For this review, take the finished solid that the model builds, in its own axes (mm). Face numbers are marked on the shaded views. A direction names the side the tool comes from. Give positions to 0.01 mm unless a question says otherwise; leave off trailing zeros. Loops run counter-clockwise (first coordinate to the right, second up) from the corner with the lowest first, then second, coordinate; pieces in that order, holes last. Notation, with made-up numbers: (47, -20) - (104, -20) arc R21 cw to (104, 10) - close; hole circle Ø3 at (15, 71.5). An arc over 180 degrees is marked (long way). Answer as CSV lines item,"result".
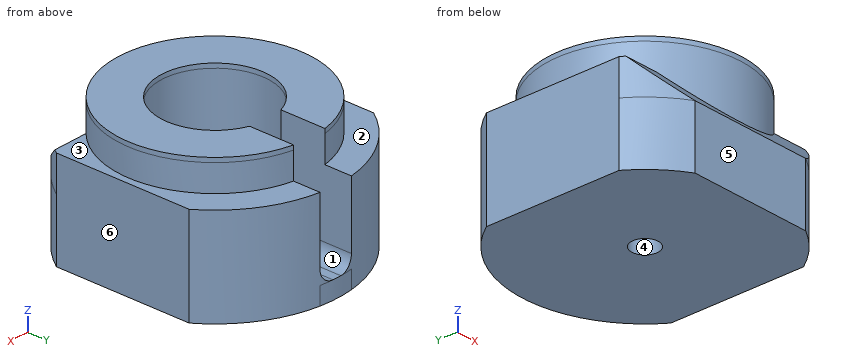
from build123d import *
from build123d.topology import SkipClean

# Parameters (mm, degrees)
SKETCH1_R               = 9.1
SKETCH1_R_2             = 6.1
BOSS_EXTRUDE1_DEPTH     = 12
BOSS_EXTRUDE2_START     = -3
SKETCH2_R               = 11
SKETCH2_R_2             = 9.1
BOSS_EXTRUDE2_DEPTH     = 3
BOSS_EXTRUDE3_START     = 4
SKETCH3_R               = 14
SKETCH3_R_2             = 11
SKETCH3_R_3             = 9.1
BOSS_EXTRUDE3_DEPTH     = 4
BOSS_EXTRUDE4_START     = 2
SKETCH4_R               = 9.1
SKETCH4_R_2             = 1.5
BOSS_EXTRUDE4_DEPTH     = 2
CUT_EXTRUDE3_DEPTH      = 23.649503306
CUT_EXTRUDE3_DEPTH_BACK = 23.649503306
SKETCH5_W               = 4
SKETCH5_H               = 12
CUT_EXTRUDE1_DEPTH      = 22.864640404
CUT_EXTRUDE4_DEPTH      = 22.864640404
CUT_EXTRUDE4_DEPTH_BACK = 22.864640404
SKETCH7_W               = 8
SKETCH7_H               = 10
BOSS_EXTRUDE5_START     = -14
SKETCH2_2_R             = 11
SKETCH2_2_R_2           = 9.1
SKETCH2_2_R_3           = 6.1
BOSS_EXTRUDE5_DEPTH     = 14
BOSS_EXTRUDE6_START     = 7
BOSS_EXTRUDE6_DEPTH     = 7
CUT_EXTRUDE5_START      = 5.762811814
CUT_EXTRUDE5_OUTLINE_W  = 4
CUT_EXTRUDE5_OUTLINE_H  = 12
CUT_EXTRUDE5_DEPTH      = 5.237188186
BOSS_EXTRUDE7_START     = -2
SKETCH11_R              = 14
SKETCH11_R_2            = 1.5
BOSS_EXTRUDE7_DEPTH     = 2
CUT_EXTRUDE6_DEPTH      = 24.151673806
CUT_EXTRUDE6_DEPTH_BACK = 24.151673806
FILLET1_R               = 1.5
BOSS_EXTRUDE8_DEPTH     = 0.5


# Read off the part's stored shape, not the designer's step: Cut-Extrude5
with BuildPart() as part:
    # Sketch1 → Boss-Extrude1 (new body)
    with BuildSketch(Plane.XY):
        Circle(SKETCH1_R)
        Circle(SKETCH1_R_2, mode=Mode.SUBTRACT)
    extrude(amount=BOSS_EXTRUDE1_DEPTH)

    # Sketch2 → Boss-Extrude2 (add)
    with BuildSketch(Plane.XY.offset(12).offset(BOSS_EXTRUDE2_START)):
        Circle(SKETCH2_R)
        Circle(SKETCH2_R_2, mode=Mode.SUBTRACT)
    extrude(amount=BOSS_EXTRUDE2_DEPTH)

    # Sketch3 → Boss-Extrude3 (add)
    # profile 1 of 2: a face of its own
    with BuildSketch(Plane(origin=(0, 0, 9), x_dir=(-1, 0, 0), z_dir=(0, 0, -1)).offset(BOSS_EXTRUDE3_START)):
        Circle(SKETCH3_R)
        with Locations(Location((0, 0, 0), (0, 0, 180))):
            Circle(SKETCH3_R_2, mode=Mode.SUBTRACT)
    # profile 2 of 2: a face of its own
    with BuildSketch(Plane(origin=(0, 0, 9), x_dir=(-1, 0, 0), z_dir=(0, 0, -1)).offset(BOSS_EXTRUDE3_START)):
        with Locations(Location((0, 0, 0), (0, 0, 180))):
            Circle(SKETCH3_R_2)
        Circle(SKETCH3_R_3, mode=Mode.SUBTRACT)
    extrude(amount=-BOSS_EXTRUDE3_DEPTH)

    # Sketch4 → Boss-Extrude4 (add)
    with BuildSketch(Plane(origin=(0, 0, 0), x_dir=(-1, 0, 0), z_dir=(0, 0, -1)).offset(BOSS_EXTRUDE4_START)):
        Circle(SKETCH4_R)
        Circle(SKETCH4_R_2, mode=Mode.SUBTRACT)
    extrude(amount=-BOSS_EXTRUDE4_DEPTH)

    # Sketch6 → Cut-Extrude3 (cut, two sides: drawn at the far end of the back side and taken through both)
    with BuildSketch(Plane.XY.offset(9).offset(-CUT_EXTRUDE3_DEPTH_BACK)):
        with BuildLine():
            ThreePointArc((11.75, -7.611668674), (14, 0), (11.75, 7.611668674))
            Line((11.75, 7.611668674), (11.75, -7.611668674))
        make_face()
        with BuildLine():
            Line((-11.75, -7.611668674), (-11.75, 7.611668674))
            ThreePointArc((-11.75, 7.611668674), (-14, 0), (-11.75, -7.611668674))
        make_face()
    extrude(amount=CUT_EXTRUDE3_DEPTH + CUT_EXTRUDE3_DEPTH_BACK, mode=Mode.SUBTRACT)

    # Sketch5 → Cut-Extrude1 (cut, through all)
    with BuildSketch(Plane(origin=(0, 0, 0), x_dir=(1, 0, 0), z_dir=(0, 1, 0))):
        with Locations((0, -6)):
            Rectangle(SKETCH5_W, SKETCH5_H)
    extrude(amount=CUT_EXTRUDE1_DEPTH, mode=Mode.SUBTRACT)

    # Sketch7 → Cut-Extrude4 (cut, two sides: drawn at the far end of the back side and taken through both)
    with BuildSketch(Plane(origin=(0, 0, 0), x_dir=(0, 0, -1), z_dir=(1, 0, 0)).offset(-CUT_EXTRUDE4_DEPTH_BACK)):
        with Locations((-8, -18.1)):
            Rectangle(SKETCH7_W, SKETCH7_H)
        Polygon((-12, -13.1), (-12, -6.1), (-12, -5.1), (-4, -13.1), align=None)
    extrude(amount=CUT_EXTRUDE4_DEPTH + CUT_EXTRUDE4_DEPTH_BACK, mode=Mode.SUBTRACT)

    # Sketch2<2> → Boss-Extrude5 (add)
    # profile 1 of 2: a face of its own
    with BuildSketch(Plane.XY.offset(12).offset(BOSS_EXTRUDE5_START)):
        Circle(SKETCH2_2_R)
        Circle(SKETCH2_2_R_2, mode=Mode.SUBTRACT)
    # profile 2 of 2: a face of its own
    with BuildSketch(Plane.XY.offset(12).offset(BOSS_EXTRUDE5_START)):
        Circle(SKETCH2_2_R_2)
        Circle(SKETCH2_2_R_3, mode=Mode.SUBTRACT)
    extrude(amount=BOSS_EXTRUDE5_DEPTH)

    # Sketch10 → Boss-Extrude6 (add)
    with BuildSketch(Plane(origin=(0, 0, 5), x_dir=(-1, 0, 0), z_dir=(0, 0, -1)).offset(BOSS_EXTRUDE6_START)):
        with BuildLine():
            Line((2, 13.856406461), (2, 10.816653826))
            ThreePointArc((2, 10.816653826), (0, -11), (-2, 10.816653826))
            Line((-2, 10.816653826), (-2, 13.856406461))
            ThreePointArc((-2, 13.856406461), (-7.550815354, 11.789197916), (-11.75, 7.611668674))
            Line((-11.75, 7.611668674), (-11.75, -7.611668674))
            ThreePointArc((-11.75, -7.611668674), (-9.660292592, -10.133052207), (-7.042016757, -12.1))
            Line((-7.042016757, -12.1), (7.042016757, -12.1))
            ThreePointArc((7.042016757, -12.1), (9.660292592, -10.133052207), (11.75, -7.611668674))
            Line((11.75, -7.611668674), (11.75, 7.611668674))
            ThreePointArc((11.75, 7.611668674), (7.550815354, 11.789197916), (2, 13.856406461))
        make_face()
    extrude(amount=-BOSS_EXTRUDE6_DEPTH)

    # Cut-Extrude5 outline → Cut-Extrude5 (cut)
    with BuildSketch(Plane(origin=(0, 0, 0), x_dir=(1, 0, 0), z_dir=(0, 1, 0)).offset(CUT_EXTRUDE5_START)):
        with Locations((0, -6)):
            Rectangle(CUT_EXTRUDE5_OUTLINE_W, CUT_EXTRUDE5_OUTLINE_H)
    extrude(amount=CUT_EXTRUDE5_DEPTH, mode=Mode.SUBTRACT)

    # Sketch11 → Boss-Extrude7 (add)
    with SkipClean():  # the faces are left unmerged after this step: merging them gives an invalid solid
        with BuildSketch(Plane.XY.offset(BOSS_EXTRUDE7_START)):
            with Locations(Location((0, 0, 0), (0, 0, 327.064769503))):
                Circle(SKETCH11_R)
            with Locations(Location((0, 0, 0), (0, 0, 180))):
                Circle(SKETCH11_R_2, mode=Mode.SUBTRACT)
        extrude(amount=BOSS_EXTRUDE7_DEPTH)

    # Sketch12 → Cut-Extrude6 (cut, two sides: drawn at the far end of the back side and taken through both)
    with SkipClean():  # the faces are left unmerged after this step: merging them gives an invalid solid
        with BuildSketch(Plane.XY.offset(-CUT_EXTRUDE6_DEPTH_BACK)):
            with BuildLine():
                Line((11.75, 7.611668674), (11.75, -7.611668674))
                ThreePointArc((11.75, -7.611668674), (14, 0), (11.75, 7.611668674))
            make_face()
            with BuildLine():
                Line((-11.75, -7.611668674), (-11.75, 7.611668674))
                ThreePointArc((-11.75, 7.611668674), (-14, 0), (-11.75, -7.611668674))
            make_face()
            with BuildLine():
                Line((7.042016757, -12.1), (-7.042016757, -12.1))
                ThreePointArc((-7.042016757, -12.1), (0, -14), (7.042016757, -12.1))
            make_face()
        extrude(amount=CUT_EXTRUDE6_DEPTH + CUT_EXTRUDE6_DEPTH_BACK, mode=Mode.SUBTRACT)

    # Fillet1
    # the kernel refuses this fillet: 1.5 mm, written as the material it adds along each edge
    with BuildSketch(Plane(origin=(-2, 2.012811814, 0), x_dir=(0, 0, 1), z_dir=(0, 1, 0))) as fillet1_piece_1_section:
        with BuildLine():
            CenterArc((FILLET1_R, FILLET1_R), FILLET1_R, 180, 90)
            Line((0, FILLET1_R), (0, 0))
            Line((0, 0), (FILLET1_R, 0))
        make_face()
    fillet1_piece_1 = extrude(amount=8.803842012, mode=Mode.PRIVATE)
    fillet1_piece_1 = fillet1_piece_1 - Plane(origin=(0, 0, 0.34289743), x_dir=(1, 0, 0), z_dir=(0, 0, -1)) * Cylinder(6.1, 24, mode=Mode.PRIVATE)
    add(fillet1_piece_1)
    with BuildSketch(Plane(origin=(2, 2.012811814, 0), x_dir=(0, 0, 1), z_dir=(0, 1, 0))) as fillet1_piece_2_section:
        with BuildLine():
            CenterArc((FILLET1_R, -FILLET1_R), FILLET1_R, 90, 90)
            Line((0, -FILLET1_R), (0, 0))
            Line((0, 0), (FILLET1_R, 0))
        make_face()
    fillet1_piece_2 = extrude(amount=8.803842012, mode=Mode.PRIVATE)
    fillet1_piece_2 = fillet1_piece_2 - Plane(origin=(0, 0, 0.342899139), x_dir=(1, 0, 0), z_dir=(0, 0, -1)) * Cylinder(6.1, 24, mode=Mode.PRIVATE)
    add(fillet1_piece_2)
    with BuildSketch(Plane(origin=(2, 10.816653826, 0), x_dir=(0, 0, 1), z_dir=(0, 1, 0))) as fillet1_piece_3_section:
        with BuildLine():
            CenterArc((FILLET1_R, -FILLET1_R), FILLET1_R, 90, 90)
            Line((0, -FILLET1_R), (0, 0))
            Line((0, 0), (FILLET1_R, 0))
        make_face()
    fillet1_piece_3 = extrude(amount=6.789752634, mode=Mode.PRIVATE)
    fillet1_piece_3 = fillet1_piece_3 & Plane(origin=(0, 0, 0.337347522), x_dir=(-1, 0, 0), z_dir=(0, 0, -1)) * Cylinder(14, 20, mode=Mode.PRIVATE)
    add(fillet1_piece_3)
    with BuildSketch(Plane(origin=(-2, 17.606406461, 0), x_dir=(0, 0, 1), z_dir=(0, -1, 0))) as fillet1_piece_4_section:
        with BuildLine():
            CenterArc((FILLET1_R, -FILLET1_R), FILLET1_R, 90, 90)
            Line((0, -FILLET1_R), (0, 0))
            Line((0, 0), (FILLET1_R, 0))
        make_face()
    fillet1_piece_4 = extrude(amount=6.789752634, mode=Mode.PRIVATE)
    fillet1_piece_4 = fillet1_piece_4 & Plane(origin=(0, 0, 0.337344923), x_dir=(-0.8392857142857146, 0.5436906195585112, 0), z_dir=(0, 0, -1)) * Cylinder(14, 20, mode=Mode.PRIVATE)
    add(fillet1_piece_4)

    # Sketch13 → Boss-Extrude8 (add)
    with BuildSketch(Plane.XY.offset(12)):
        with BuildLine():
            Line((-2, 5.762811814), (-2, 10.816653826))
            ThreePointArc((-2, 10.816653826), (0, -11), (2, 10.816653826))
            Line((2, 10.816653826), (2, 5.762811814))
            ThreePointArc((2, 5.762811814), (0, -6.1), (-2, 5.762811814))
        make_face()
    extrude(amount=BOSS_EXTRUDE8_DEPTH)


solid = part.part
1) Consider section D-D on z = 0.5. Write out the cut boundary in (x, y).
From the geometry:
outline,"(-11.75, -7.61) arc R14 ccw to (-7.04, -12.1) - (7.04, -12.1) arc R14 ccw to (11.75, -7.61) - (11.75, 7.61) arc R14 ccw to (1.62, 13.91) - (1.62, 5.88) arc R6.1 cw (long way) to (-1.62, 5.88) - (-1.62, 13.91) arc R14 ccw to (-11.75, 7.61) - close"
2) Consider section B-B on y = 0. Write out the cut boundary in (x, z), and give its area (3 significant figures).
From the geometry:
outline,"(-11.75, -2) - (-1.5, -2) - (-1.5, 0) - (-6.1, 0) - (-6.1, 12.5) - (-11, 12.5) - (-11, 9) - (-11.75, 9) - close; (1.5, -2) - (11.75, -2) - (11.75, 9) - (11, 9) - (11, 12.5) - (6.1, 12.5) - (6.1, 0) - (1.5, 0) - close"
area,"177 mm^2"
3) Wall thickness on line 1 (Y direction, x = 0, z = -1.25); line 2 (X direction, y = 0, z = 3.5); line 3 (X direction, y = 0, z = 12.25): over which ranges is each line inside the solid? List them lowest first. Write a range as from..to.
From the geometry:
line 1,"y = -12.1..-1.5, 1.5..14"
line 2,"x = -11.75..-6.1, 6.1..11.75"
line 3,"x = -11..-6.1, 6.1..11"
4) Draft analysis for pull direction Y (two halves, no side actions). For the marked faces 4, 5 and 6, state which applies: pulls with the +Y half, pulls with the -Y half, needs draft (parallel to the pull), parting line crosses it, or undercut.
From the geometry:
face 4,"undercut"
face 5,"pulls with the -Y half"
face 6,"needs draft"
5) Machinability: for the marked faces 1, 2 and 3, which of the approach directions +Z, -Z, +X, -X, +Y, -Y give a long, thin tool a straight path to every point of the face, cutting with its end or side? Answer none if there is none.
From the geometry:
face 1,"+Z, +Y"
face 2,"+Z, -X"
face 3,"+Z, +X"
6) Consider section C-C on x = -5. Write out the cut boundary in (y, z), and give its area (3 significant figures).
From the geometry:
outline,"(-12.1, -2) - (13.08, -2) - (13.08, 9) - (9.8, 9) - (9.8, 12.5) - (3.49, 12.5) - (3.49, 0) - (-3.49, 0) - (-3.49, 12.5) - (-9.8, 12.5) - (-9.8, 7.3) - (-12.1, 5) - close"
area,"252 mm^2"
7) Insertion check: P1, Ø3, axis at x = 3, z = 5, coming from the +Y side. The pin has a flat end and moves straight along its axis. Give the tip position at first contact, or say it passes through.
From the geometry:
P1,"stops at y = 13.86"
8) Consider section A-A on x = 0. Write out the cut boundary in (y, z).
From the geometry:
outline,"(-12.1, -2) - (-1.5, -2) - (-1.5, 0) - (-6.1, 0) - (-6.1, 12.5) - (-11, 12.5) - (-11, 6.1) - (-12.1, 5) - close; (1.5, -2) - (14, -2) - (14, 0) - (1.5, 0) - close"
